Autodesk Inventor part; units mm, degrees
ref_plane "YZ Plane" through (0, 0, 0) normal (1, 0, 0) x (0, 1, 0)
ref_plane "XZ Plane" through (0, 0, 0) normal (0, 1, 0) x (-1, 0, 0)
ref_plane "XY Plane" through (0, 0, 0) normal (0, 0, 1) x (1, 0, 0)
sketch "Skizze1" plane through (0, 0, 0) normal (0, 0, 1) x (1, 0, 0)
  line L0 (40, 40) -> (40, -40)
  line L1 (40, -40) -> (-40, -40)
  line L2 (-40, -40) -> (-40, 40)
  line L3 (-40, 40) -> (40, -40) construction
  line L4 (40, 40) -> (-40, -40) construction
  line L5 (-20, 40) -> (-20, -20)
  line L6 (-20, -20) -> (20, -20)
  line L7 (20, -20) -> (20, 40)
  line L8 (-40, 40) -> (-20, 40)
  line L9 (20, 40) -> (40, 40)
  point P0 (0, 0)
  dimension "d0" = 40
  dimension "d1" = 80
extrude "Extrusion1" add sketch "Skizze1" along normal blind 10
sketch "Skizze2" plane through (0, 0, 10) normal (0, 0, 1) x (1, 0, 0)
  line L0 (-40, 40) -> (-40, -40)
  line L1 (40, 40) -> (20, 40)
  line L2 (20, 40) -> (20, -20)
  line L3 (20, -20) -> (-20, -20)
  line L4 (-20, -20) -> (-20, 40)
  line L5 (-20, 40) -> (-40, 40)
  line L6 (-25, 40) -> (-25, -20.7574)
  line L7 (-20.7574, -25) -> (20.7574, -25)
  line L8 (25, -20.7574) -> (25, 40)
  arc A0 (20.7574, -25) -> (25, -20.7574) centre (22.8787, -22.8787) ccw
  arc A1 (-25, -20.7574) -> (-20.7574, -25) centre (-22.8787, -22.8787) ccw
  line L9 (0, 56) -> (0, -56) construction
  point P0 (0, 0)
  dimension "d5" = 6
  dimension "d7" = 2.1213
  dimension "d8" = 2.1213
  dimension "d9" = 50
  dimension "d11" = 5
  dimension "d12" = 5
extrude "Extrusion2" cut sketch "Skizze2" against normal blind 6
fillet "Rundung1" radius 3 2 edges at (20, -20, 2) (-20, -20, 2)
chamfer "Fase1" distance 10 angle 45 2 edges at (-20, 40, 2) (20, 40, 2)
sketch "Skizze3" plane through (0, 0, 0) normal (0, 0, -1) x (-1, 0, 0)
  line L0 (-40, 40) -> (-20, 40)
  line L1 (-40, -40) -> (-40, 40)
  line L2 (40, -40) -> (-40, -40)
  line L3 (40, 40) -> (40, -40)
  line L4 (35, -35) -> (-35, -35)
  line L5 (-35, -35) -> (-35, 35)
  line L6 (-35, 35) -> (35, 35)
  line L7 (35, 35) -> (35, -35)
  line L8 (35, -35) -> (-35, 35) construction
  line L9 (-35, -35) -> (35, 35) construction
  point P0 (-21, 40)
  point P1 (0, 0)
  point P2 (0, 0)
  dimension "d22" = 5
  dimension "d23" = 5
  dimension "d24" = 5
  dimension "d25" = 5
  dimension "d33" = 70
  dimension "d34" = 70
hole "Bohrung1" at (-35, 35, 0) at (-35, -35, 0) at (35, -35, 0) at (35, 35, 0) direction (0, 0, 1) diameter 4.5 end through all countersink diameter 10 countersink angle 90
equation "\"d8\" = d7"
equation "\"d12\" = d11"
equation "\"d23\" = d22"
equation "\"d24\" = d22"
equation "\"d25\" = d22"
properties part number "Tunel_OdourPortSlidingMechanism" material "Polycarbonat, klar"
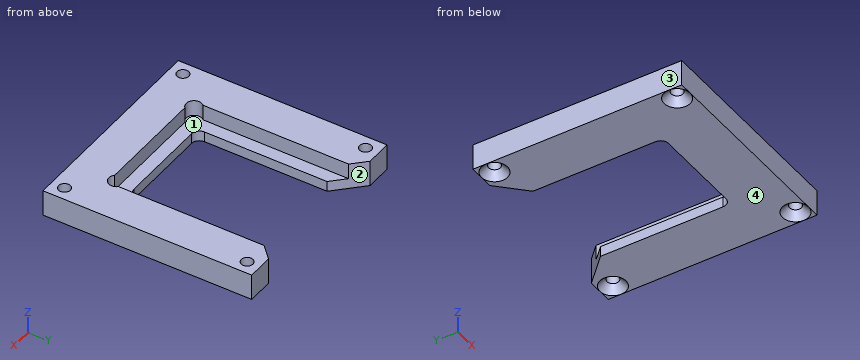
Can you work these out from the model? Positions are in its coordinate system, mm. Face numbers are marked on the shaded views. Give positions to 0.01 mm unless a question says otherwise; leave off trailing zeros. Order: outer loops, then holes, each group sorted by start corner. A loop starts at its lowest first (then second) coordinate and runs counter-clockwise, first axis right, second up. Notation, with made-up numbers: (60, -36) - (96, -36) arc R31 ccw to (96, -11) - close; hole circle Ø7 at (-40, -37.5). An arc over 180 degrees is marked (long way). Use a Markdown table: item, result. Add a question column.
Q1. If we section it at C-C on x = 7: Write out the boundary of the cut face in (y, z).
Q2. If we section it at D-D on z = 1.25: Write out the boundary of the cut face in (x, y), plus the area to 3 significant figures.
Q3. If we section it at B-B on y = 7.5: Write out the boundary of the cut face in (x, z).
Q4. Please list where these lines run through material, in increasing order: line 1 along Y through (x, z) = (35, 8.5); line 2 along X through (y, z) = (35, 7.25).
Q5. If we mould it in two halves opening along X, with no side actions, what happens to the marked faces 1, 2, 3 and 4? For each: released by +X, released by -X, zero draft, split by the parting line, or undercut.
Q6. I'm going to push flat-ended pins straight in: pin 1 (4.5 mm diameter, centred on x = 2, z = 2.5, fed in from +Y); pin 2 (1.8 mm diameter, centred on x = -10.5, z = 6, fed in from +Y); pin 3 (1 mm diameter, centred on x = -21, z = 2, fed in from +Y). Where does each tip first touch, or does it pass through?
Q7. If we section it at A-A on z = 7.5: Write out the boundary of the cut face in (x, y), plus the area to 3 significant figures.
Answers follow:
| question | item | result |
|---|---|---|
| 1 | outline | (-40, 0) - (-20, 0) - (-20, 4) - (-25, 4) - (-25, 10) - (-40, 10) - close |
| 2 | outline | (-40, -40) - (40, -40) - (40, 40) - (30, 40) - (20, 30) - (20, -17) arc R3 cw to (17, -20) - (-17, -20) arc R3 cw to (-20, -17) - (-20, 30) - (-30, 40) - (-40, 40) - close; hole circle Ø7.5 at (-35, -35); hole circle Ø7.5 at (-35, 35); hole circle Ø7.5 at (35, -35); hole circle Ø7.5 at (35, 35) |
| 2 | area | 3,730 mm^2 |
| 3 | outline | (-40, 0) - (-20, 0) - (-20, 4) - (-25, 4) - (-25, 10) - (-40, 10) - close; (20, 0) - (40, 0) - (40, 10) - (25, 10) - (25, 4) - (20, 4) - close |
| 4 | line 1 | y = -40 to -37.25, -32.75 to 32.75, 37.25 to 40 |
| 4 | line 2 | x = -40 to -37.25, -32.75 to -25, 25 to 32.75, 37.25 to 40 |
| 5 | face 1 | undercut |
| 5 | face 2 | undercut |
| 5 | face 3 | released by -X |
| 5 | face 4 | zero draft |
| 6 | pin 1 | stops at y = -20 |
| 6 | pin 2 | stops at y = -25 |
| 6 | pin 3 | stops at y = 31.5 |
| 7 | outline | (-40, -40) - (40, -40) - (40, 40) - (30, 40) - (25, 35) - (25, -20.76) arc R3 cw to (20.76, -25) - (-20.76, -25) arc R3 cw to (-25, -20.76) - (-25, 35) - (-30, 40) - (-40, 40) - close; hole circle Ø4.5 at (-35, -35); hole circle Ø4.5 at (-35, 35); hole circle Ø4.5 at (35, -35); hole circle Ø4.5 at (35, 35) |
| 7 | area | 3,050 mm^2 |
